from build123d import *

# Parameters (mm, degrees)
BOSS_EXTRUDE1_DEPTH = 20
SKETCH2_W           = 150
SKETCH2_H           = 65
BOSS_EXTRUDE2_DEPTH = 97
SKETCH4_W           = 100
SKETCH4_H           = 80
BOSS_EXTRUDE3_DEPTH = 22
SKETCH5_W           = 90
SKETCH5_H           = 60
BOSS_EXTRUDE4_DEPTH = 20
SKETCH7_W           = 75
SKETCH7_H           = 55
BOSS_EXTRUDE5_DEPTH = 18
SKETCH9_W           = 50
SKETCH9_H           = 50
BOSS_EXTRUDE6_DEPTH = 30
SKETCH10_R          = 10
BOSS_EXTRUDE7_DEPTH = 40


with BuildPart() as part:
    # Sketch1 → Boss-Extrude1 (new body)
    with BuildSketch(Plane(origin=(0, 0, 0), x_dir=(1, 0, 0), z_dir=(0, 1, 0))):
        with BuildLine():
            Line((-122.288467544, 114.797617793), (122.288467544, 114.797617793))
            ThreePointArc((122.288467544, 114.797617793), (145.765834901, 103.474159817), (151.520203415, 78.051832592))
            Line((151.520203415, 78.051832592), (105.366357261, -121.948167408))
            ThreePointArc((105.366357261, -121.948167408), (94.811163415, -138.679749564), (76.13462139, -145.202382207))
            Line((76.13462139, -145.202382207), (-76.13462139, -145.202382207))
            ThreePointArc((-76.13462139, -145.202382207), (-94.811163415, -138.679749564), (-105.366357261, -121.948167408))
            Line((-105.366357261, -121.948167408), (-151.520203415, 78.051832592))
            ThreePointArc((-151.520203415, 78.051832592), (-145.765834901, 103.474159817), (-122.288467544, 114.797617793))
        make_face()
    extrude(amount=-BOSS_EXTRUDE1_DEPTH)

    # Sketch2 → Boss-Extrude2 (add)
    with BuildSketch(Plane(origin=(0, 0, 0), x_dir=(1, 0, 0), z_dir=(0, 1, 0))):
        with Locations((-59.803637432, 70.737817799)):
            Rectangle(SKETCH2_W, SKETCH2_H)
    extrude(amount=BOSS_EXTRUDE2_DEPTH)

    # Sketch4 → Boss-Extrude3 (add)
    with BuildSketch(Plane(origin=(0, 0, 0), x_dir=(1, 0, 0), z_dir=(0, 1, 0))):
        with Locations((73.379228632, 61.908908542)):
            Rectangle(SKETCH4_W, SKETCH4_H)
    extrude(amount=BOSS_EXTRUDE3_DEPTH)

    # Sketch5 → Boss-Extrude4 (add)
    with BuildSketch(Plane(origin=(0, 22, 0), x_dir=(1, 0, 0), z_dir=(0, 1, 0))):
        with Locations((73.353532596, 63.452591803)):
            Rectangle(SKETCH5_W, SKETCH5_H)
    extrude(amount=BOSS_EXTRUDE4_DEPTH)

    # Sketch7 → Boss-Extrude5 (add)
    with BuildSketch(Plane(origin=(0, 0, 0), x_dir=(1, 0, 0), z_dir=(0, 1, 0))):
        with Locations((-80.583724221, 1.784070664)):
            Rectangle(SKETCH7_W, SKETCH7_H)
    extrude(amount=BOSS_EXTRUDE5_DEPTH)

    # Sketch9 → Boss-Extrude6 (add)
    with BuildSketch(Plane(origin=(0, 0, 0), x_dir=(1, 0, 0), z_dir=(0, 1, 0))):
        with Locations((-9.322697354, 0.802057889)):
            Rectangle(SKETCH9_W, SKETCH9_H)
    extrude(amount=BOSS_EXTRUDE6_DEPTH)

    # Sketch10 → Boss-Extrude7 (add)
    with BuildSketch(Plane(origin=(-126.757825315, 0, 29.251805842), x_dir=(0.224859507, 0, 0.974391196), z_dir=(-0.974391196, 0, 0.224859507))):
        with Locations((80.281358312, -9.946535293)):
            Circle(SKETCH10_R)
        with Locations((-98.316139362, -9.946535293)):
            Circle(SKETCH10_R)
    boss_extrude7 = extrude(amount=BOSS_EXTRUDE7_DEPTH)

    # Mirror6: Boss-Extrude7 across plane
    add(boss_extrude7.mirror(Plane(origin=(0, 0, 0), x_dir=(0, 0, 1), z_dir=(1, 0, 0))))


solid = part.part
Input: part model. Units: mm. Frame: model coordinates. A direction names the side the tool comes from. Coordinates: 2 decimals unless noted, no trailing zeros. Loops run counter-clockwise (first coordinate to the right, second up) from the corner with the lowest first, then second, coordinate; pieces in that order, holes last.
Q1. Draft query along X for faces 6 (the face through (-147.71, -9.81, 116.34)), 7 (the face through (-81, 9, -29.284)), 8 (the face through (165.94, -6.94, -52.82)), 9 (the face through (147.71, -9.81, 116.34)). Return one class per face: +X half, -X half, draft (parallel to the pull), parting line (faces both ways), or undercut.
Q2. Contact query for flat-ended pins moving along their axis: pin 1 (17.5 mm diameter, centred on y = 12, z = -53, fed in from -X); pin 2 (10 mm diameter, centred on y = 5.5, z = 113.5, fed in from -X); pin 3 (16 mm diameter, centred on y = 27, z = -77.5, fed in from +X); pin 4 (15 mm diameter, centred on x = -2, y = 9, fed in from -Z). Output: stop coordinate, or through.
Q3. Cut plane D-D (z = 70.5). Output: boundary loops of the cut face in (x, y).
Q4. Material intervals for line 1 (X direction, y = 30.5, z = -82.5); line 2 (Z direction, x = -106, y = 4); line 3 (X direction, y = 14.5, z = 24.5), sorted ascending.
Q5. Set-up query: faces 1 (the face through (-61, 48, -38.238)), 2 (the face through (-61, 48, -103.238)), 3 (the face through (73, 32, -33.453)), 4 (the face through (73, 11, -101.909)), 5 (the face through (73, 42, -64)). Return all of +Z, -Z, +X, -X, +Y, -Y with unobstructed straight access to the full face (end or side cutting, diameter ignored); none if empty.
Q6. Cut plane B-B (z = 11). Output: boundary loops of the cut face in (x, y), then the cut area to 3 significant figures.
Q7. Cut plane C-C (y = 48.5). Output: boundary loops of the cut face in (x, z), then the cut area to 3 significant figures.
Q8. Cut plane A-A (x = 72). Output: boundary loops of the cut face in (y, z), then the cut area to 3 significant figures.
Working result:
1. face 6: -X half
1. face 7: draft
1. face 8: undercut
1. face 9: +X half
2. pin 1: stops at x = -134.8
2. pin 2: passes through
2. pin 3: stops at x = 123.38
2. pin 4: stops at z = -103.24
3. outline: (-117.24, -20) - (117.24, -20) - (117.24, 0) - (-117.24, 0) - close
4. line 1: x = -134.8 to 15.2, 28.35 to 118.35
4. line 2: z = -103.24 to -38.24, -29.28 to 25.72
4. line 3: x = -118.08 to -43.08
5. face 1: -X, +Y
5. face 2: -Z, +X, -X, +Y
5. face 3: +Z, +X, -X, +Y
5. face 4: -Z, +X, +Y
5. face 5: +Z, -Z, +X, +Y
6. outline: (-130.97, -20) - (130.97, -20) - (130.97, 0) - (15.68, 0) - (15.68, 30) - (-34.32, 30) - (-34.32, 0) - (-43.08, 0) - (-43.08, 18) - (-118.08, 18) - (-118.08, 0) - (-130.97, 0) - close
6. area: 8,090 mm2
7. outline: (-134.8, -103.24) - (15.2, -103.24) - (15.2, -38.24) - (-134.8, -38.24) - close
7. area: 9,750 mm2
8. outline: (-20, -114.8) - (0, -114.8) - (0, -101.91) - (22, -101.91) - (22, -93.45) - (42, -93.45) - (42, -33.45) - (22, -33.45) - (22, -21.91) - (0, -21.91) - (0, 145.2) - (-20, 145.2) - close
8. area: 8,160 mm2
